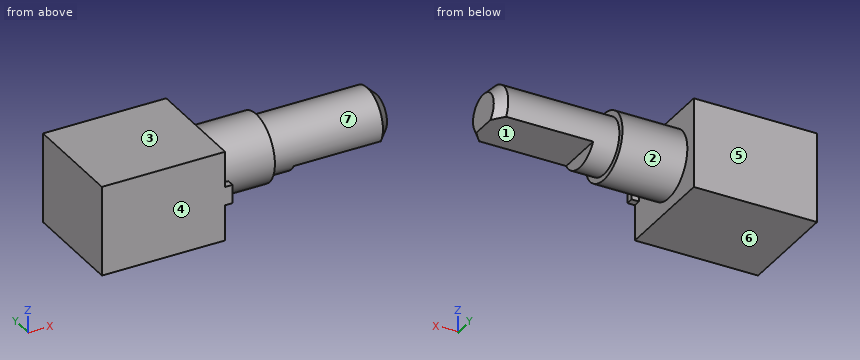
```python
from build123d import *

# Parameters (mm, degrees)
SKETCH1_W           = 13.3
SKETCH1_H           = 11.35
BOSS_EXTRUDE1_DEPTH = 9.7
SKETCH2_R           = 3.6
BOSS_EXTRUDE2_DEPTH = 7
SKETCH3_R           = 3
BOSS_EXTRUDE4_DEPTH = 13
SKETCH4_W           = 2
SKETCH4_H           = 0.8
BOSS_EXTRUDE5_DEPTH = 0.8
SKETCH5_W           = 9.645805708
SKETCH5_H           = 9.062919638
CUT_EXTRUDE1_DEPTH  = 10.4
CHAMFER1_SIZE       = 1


with BuildPart() as part:
    # Sketch1 → Boss-Extrude1 (new body)
    with BuildSketch(Plane.XY):
        with Locations((6.65, 5.675)):
            Rectangle(SKETCH1_W, SKETCH1_H)
    extrude(amount=BOSS_EXTRUDE1_DEPTH)

    # Sketch2 → Boss-Extrude2 (add)
    with BuildSketch(Plane(origin=(13.3, 0, 0), x_dir=(0, 0, -1), z_dir=(1, 0, 0))):
        with Locations(Location((-4.85, 6.5, 0), (0, 0, 270))):  # turned: the seam where the file's is
            Circle(SKETCH2_R)
    extrude(amount=BOSS_EXTRUDE2_DEPTH)

    # Sketch3 → Boss-Extrude4 (add)
    with BuildSketch(Plane(origin=(20.3, 0, 0), x_dir=(0, 0, -1), z_dir=(1, 0, 0))):
        with Locations(Location((-4.85, 6.5, 0), (0, 0, 270))):  # turned: the seam where the file's is
            Circle(SKETCH3_R)
    extrude(amount=BOSS_EXTRUDE4_DEPTH)

    # Sketch4 → Boss-Extrude5 (add)
    with BuildSketch(Plane(origin=(13.3, 0, 0), x_dir=(0, 0, -1), z_dir=(1, 0, 0))):
        with Locations((-4.85, 0.4)):
            Rectangle(SKETCH4_W, SKETCH4_H)
    extrude(amount=BOSS_EXTRUDE5_DEPTH)

    # Sketch5 → Cut-Extrude1 (cut)
    with BuildSketch(Plane(origin=(33.3, 0, 0), x_dir=(0, 0, -1), z_dir=(1, 0, 0))):
        with Locations((1.472902854, 6.5)):
            Rectangle(SKETCH5_W, SKETCH5_H)
    extrude(amount=-CUT_EXTRUDE1_DEPTH, mode=Mode.SUBTRACT)

    # Chamfer1
    chamfer1_edges = [part.edges().sort_by_distance(p)[0] for p in [
        (33.3, 7.276457135, 7.747777479),
    ]]
    chamfer(chamfer1_edges, length=CHAMFER1_SIZE)


solid = part.part
```
Work out the finished part from the listing and answer in its coordinate system (mm). Face numbers are marked on the shaded views. A direction names the side the tool comes from. Give positions to 0.01 mm unless a question says otherwise; leave off trailing zeros. Write each loop counter-clockwise with the first axis right and the second up, starting at its lowest first coordinate (ties: lowest second). Pieces come first, ordered by that corner, then holes. Notation, with made-up numbers: (-24, 32.25) -> (3, 32.25) arc R16 cw to (3, 50.25) -> close; hole circle Ø3 at (81.25, -30). An arc over 180 degrees is marked (long way). Write item = value, one per line.
Q1. Section C-C on x = 29.5 is taken. Determine the outline of the cut face in (y, z), and give its area (3 significant figures).
Computed values:
outline = (3.9, 3.35) -> (9.1, 3.35) arc R3 ccw (long way) to start
area = 22.7 mm^2
Q2. Section A-A on z = 4.85 is taken. Determine the outline of the cut face in (x, y), and give its area (3 significant figures).
Computed values:
outline = (0, 0) -> (14.1, 0) -> (14.1, 0.8) -> (13.3, 0.8) -> (13.3, 2.9) -> (20.3, 2.9) -> (20.3, 3.5) -> (32.3, 3.5) -> (33.3, 4.5) -> (33.3, 8.5) -> (32.3, 9.5) -> (20.3, 9.5) -> (20.3, 10.1) -> (13.3, 10.1) -> (13.3, 11.35) -> (0, 11.35) -> close
area = 279 mm^2
Q3. Consider line 1 along X through (y, z) = (1, 7.25); line 2 along Y through (x, z) = (16, 5); line 3 along Y through (x, z) = (29, 3.5). Determine where each line is inside the solid, lowest interval first.
Computed values:
line_1 = 0 to 13.3
line_2 = 2.9 to 10.1
line_3 = 3.82 to 9.18
Q4. Section B-B on y = 6.5 is taken. Determine the outline of the cut face in (x, z).
Computed values:
outline = (0, 0) -> (13.3, 0) -> (13.3, 1.25) -> (20.3, 1.25) -> (20.3, 1.85) -> (22.9, 1.85) -> (22.9, 3.35) -> (33.3, 3.35) -> (33.3, 6.85) -> (32.3, 7.85) -> (20.3, 7.85) -> (20.3, 8.45) -> (13.3, 8.45) -> (13.3, 9.7) -> (0, 9.7) -> close
Q5. Flat-ended cylindrical pins translate along their axes: pin 1 Ø0.9 at (x, y) = (13.5, 0.5) entering from -Z; pin 2 Ø4 at (x, y) = (28.5, 5.5) entering from +Z; pin 3 Ø4 at (x, y) = (22, 8) entering from +Z; pin 4 Ø5.5 at (x, y) = (29.5, 6.5) entering from -Z. Find the tip coordinate at first contact, or state that the pin passes through.
Computed values:
pin_1 = 0
pin_2 = 7.85
pin_3 = 8.42
pin_4 = 3.35
Q6. A tool of negligible diameter and unlimited length cuts with its end or side. For the marked faces 1, 2 and 3, from which of +Z, -Z, +X, -X, +Y, -Y can it reach the whole face along a straight path? Write none if from no direction.
Computed values:
face_1 = -Z, +X, +Y, -Y
face_2 = +X
face_3 = +Z, +X, -X, +Y, -Y
Q7. Section D-D on y = 1.5 is taken. Determine the outline of the cut face in (x, z).
Computed values:
outline = (0, 0) -> (13.3, 0) -> (13.3, 9.7) -> (0, 9.7) -> close
Q8. For a pull along Y with two mould halves and no side action, classify the marked faces 4, 5, 6 and 7 as pulls with the +Y half, pulls with the -Y half, needs draft (parallel to the pull), parting line crosses it, or undercut.
Computed values:
face_4 = pulls with the -Y half
face_5 = pulls with the +Y half
face_6 = needs draft
face_7 = parting line crosses it
